For this review, take the finished solid that the model builds, in its own axes (mm). A direction names the side the tool comes from. Give positions to 0.01 mm unless a question says otherwise; leave off trailing zeros. Order: outer loops, then holes, each group sorted by start corner. A loop starts at its lowest first (then second) coordinate and runs counter-clockwise, first axis right, second up. Notation, with made-up numbers: (8.25, 54) - (60.25, 54) arc R18 ccw to (60.25, 87) - close; hole circle Ø5 at (3.25, -40). An arc over 180 degrees is marked (long way). Put each result on its own line as item: value. Start each with the question number.
Autodesk Inventor part; units mm, degrees
ref_plane "Work Plane1" through (0, 4.0415, 15) normal (1, 0, 0) x (0, 1, 0)
ref_plane "YZ Plane" through (0, 0, 0) normal (1, 0, 0) x (0, 1, 0)
ref_plane "XZ Plane" through (0, 0, 0) normal (0, 1, 0) x (-1, 0, 0)
sketch "Sketch1" plane through (0, 0, 0) normal (0, 0, 1) x (1, 0, 0)
  circle A0 centre (0, 0) radius 3
  dimension "d0" = 6
extrude "Extrusion1" add sketch "Sketch1" along normal blind 12
sketch "Sketch2" plane through (0, 0, 12) normal (0, 0, 1) x (1, 0, 0)
  line L0 (3.5, -2.0207) -> (0, -4.0415)
  line L1 (0, -4.0415) -> (-3.5, -2.0207)
  line L2 (-3.5, -2.0207) -> (-3.5, 2.0207)
  line L3 (-3.5, 2.0207) -> (0, 4.0415)
  line L4 (0, 4.0415) -> (3.5, 2.0207)
  line L5 (3.5, 2.0207) -> (3.5, -2.0207)
  point P0 (0, 0)
  point P1 (0, 0)
  dimension "d3" = 7
extrude "Extrusion2" add sketch "Sketch2" along normal blind 3
sketch "Sketch3" plane through (3.5, -2.0207, 12) normal (1, 0, 0) x (0, 0, -1)
  line L0 (12, 2.0207) -> (-9.0637, 2.0207) construction
  line L1 (-5, 2.0207) -> (-3, 3.7707)
  line L2 (-3, 0) -> (-3, 4.0415)
  dimension "d6" = 2
  dimension "d7" = 1.75
ref_plane "Work Plane1" through (0, 4.0415, 15) normal (1, 0, 0) x (0, 1, 0)
sketch "Sketch4" plane through (0, 4.0415, 15) normal (1, 0, 0) x (0, 1, 0)
  line L0 (-4.0415, -15) -> (-4.0415, 0)
  line L1 (-4.0415, 2) -> (-2.2915, 0)
  line L2 (-6.0622, 0) -> (-2.0207, 0)
  line L3 (-4.0415, 2) -> (-4.0415, 9.3092)
  line L4 (-4.0415, 0) -> (-4.0415, 2)
  line L5 (-2.2915, 0) -> (-4.0415, 0)
  dimension "d8" = 1.75
  dimension "d9" = 2
revolve "Revolution1" add sketch "Sketch4" angle 360 about axis through (0, 0, 17) along (0, 0, 1)
sketch "Sketch5" plane through (0, 0, 0) normal (0, 0, -1) x (-1, 0, 0)
  circle A0 centre (0, 0) radius 0.875
  dimension "d11" = 1.75
extrude "Extrusion3" cut sketch "Sketch5" against normal blind 15
sketch "Sketch6" plane through (0, 0, 15) normal (0, 0, -1) x (-1, 0, 0)
  circle A0 centre (0, 0) radius 0.2
  dimension "d14" = 0.4
extrude "Extrusion4" cut sketch "Sketch6" against normal through all
thread "Thread1"
properties part number "nozzle"
1. Add section A-A, the plane y = 0. Give the boundary of the cut face in (x, z) (3 decimals).
2. Clearance check with flat-ended pins moving along their axes: pin 1 (2 mm diameter, centred on x = -2.5, z = 12.5, fed in from +Y); pin 2 (1.5 mm diameter, centred on y = -2, z = 6, fed in from +X); pin 3 (1.6 mm diameter, centred on x = 0, y = 0, fed in from -Z). State where each tip first meets the part, or that it passes through.
3. Tool access review of faces 5 (the face through (-1, -3, 12)), 6 (the face through (-3.5, 0, 13)), 7 (the face through (-2, -1, 15)): name each direction out of +Z, -Z, +X, -X, +Y, -Y from which nothing blocks a thin tool from reaching the whole face with its end or side.
4. Add section C-C, the plane z = 11.25. Give the boundary of the cut face in (x, y) (3 decimals), then the cut area to 3 significant figures.
5. Add section D-D, the plane y = -2.75. Give the boundary of the cut face in (x, z), then the cut area to 3 significant figures.
6. Wall thickness on line 1 (Y direction, x = 0, z = 4) (3 decimals); line 2 (Z direction, x = 1, y = 2.25); line 3 (X direction, y = -0.75, z = 10.5): over which ranges is each line inside the solid? List them lowest first. Write a range as from..to.
7. The part is to be moulded in two halves that separate along Y. For faces 1 (the face through (-3, 0, 6)), 2 (the face through (-0.808, -0.335, 7.395)), 3 (the face through (1.726, 3.045, 13.479)), 4 (the face through (3.5, 0, 13)), say which applies: released by +Y, released by -Y, zero draft, split by the parting line, or undercut.
8. Add section B-B, the plane x = 2. Give the boundary of the cut face in (y, z), then the cut area to 3 significant figures.
Found:
1. outline: (-3.5, 12) - (-3, 12) - (-3, 0) - (-0.875, 0) - (-0.875, 15) - (-0.2, 15) - (-0.2, 16.771) - (-1.75, 15) - (-3.5, 15) - close; (0.2, 15) - (0.875, 15) - (0.875, 0) - (3, 0) - (3, 12) - (3.5, 12) - (3.5, 15) - (1.75, 15) - (0.2, 16.771) - close
2. pin 1: stops at y = 3.18
2. pin 2: stops at x = 2.73
2. pin 3: stops at z = 15
3. face 5: -Z
3. face 6: +Z, -Z, -X, +Y, -Y
3. face 7: +Z
4. outline: circle Ø6 at (0, 0); hole circle Ø1.75 at (0, 0)
4. area: 25.9 mm^2
5. outline: (-2.24, 12) - (-1.2, 12) - (-1.2, 0) - (1.2, 0) - (1.2, 12) - (2.24, 12) - (2.24, 15) - (-2.24, 15) - close
5. area: 42.2 mm^2
6. line 1: y = -3..-0.875, 0.875..3
6. line 2: z = 0..15
6. line 3: x = -2.9..-0.45, 0.45..2.9
7. face 1: split by the parting line
7. face 2: undercut
7. face 3: released by +Y
7. face 4: zero draft
8. outline: (-2.89, 12) - (-2.24, 12) - (-2.24, 0) - (2.24, 0) - (2.24, 12) - (2.89, 12) - (2.89, 15) - (-2.89, 15) - close
8. area: 71.0 mm^2
